Source: CAD feature listing. Evaluate the final solid. Frame: model axes, mm. A direction names the side the tool comes from. Give positions to 0.01 mm unless a question says otherwise; leave off trailing zeros. Loops run counter-clockwise (first coordinate to the right, second up) from the corner with the lowest first, then second, coordinate; pieces in that order, holes last.
Autodesk Inventor part; units mm, degrees
ref_plane "YZ Plane" through (0, 0, 0) normal (1, 0, 0) x (0, 1, 0)
ref_plane "XZ Plane" through (0, 0, 0) normal (0, 1, 0) x (-1, 0, 0)
ref_plane "XY Plane" through (0, 0, 0) normal (0, 0, 1) x (1, 0, 0)
sketch "Esboço1" plane through (0, 0, 0) normal (0, 0, 1) x (1, 0, 0)
  line L0 (0, 0) -> (44, 0)
  line L1 (44, 0) -> (44, 50)
  line L2 (44, 50) -> (0, 50)
  line L3 (0, 50) -> (0, 0)
  dimension "d0" = 44
  dimension "d1" = 50
extrude "Extrusão1" add sketch "Esboço1" along normal blind 3
sketch "Esboço2" plane through (0, 0, 0) normal (-1, 0, 0) x (0, 0, 1)
  line L0 (0, 0) -> (0, 50)
  line L1 (0, 50) -> (-16, 50)
  line L2 (-16, 50) -> (-16, 0)
  line L3 (-16, 0) -> (0, 0)
  line L4 (0, 0) -> (0, 50)
  line L5 (0, 50) -> (-8, 50) construction
  line L6 (-8, 50) -> (-8, 42) construction
  line L7 (0, 0) -> (-8, 0) construction
  line L8 (-8, 0) -> (-8, 8) construction
  circle A0 centre (-8, 42) radius 3
  circle A1 centre (-8, 8) radius 3
  dimension "d4" = 16
  dimension "d5" = 50
  dimension "d6" = 8
  dimension "d7" = 8
  dimension "d8" = 8
  dimension "d9" = 8
  dimension "d10" = 6
  dimension "d11" = 6
extrude "Extrusão2" add sketch "Esboço2" against normal blind 3
sketch "Esboço3" plane through (44, 0, 0) normal (1, 0, 0) x (0, 0, -1)
  line L0 (0, 50) -> (-3, 50)
  line L1 (-3, 50) -> (46, 50)
  line L2 (46, 50) -> (46, 0)
  line L3 (46, 0) -> (-3, 0)
  line L4 (-3, 0) -> (-3, 50)
  point P0 (0, 0)
  dimension "d14" = 49
extrude "Extrusão3" add sketch "Esboço3" along normal blind 3
sketch "Esboço4" plane through (44, 0, -46) normal (0, 0, -1) x (-1, 0, 0)
  line L0 (0, 50) -> (41, 50) construction
  line L1 (0, 50) -> (8, 50) construction
  line L2 (8, 50) -> (8, 42) construction
  line L3 (0, 50) -> (0, 0) construction
  line L4 (0, 0) -> (8, 0) construction
  line L5 (41, 0) -> (0, 0) construction
  line L6 (8, 0) -> (8, 8) construction
  circle A0 centre (8, 42) radius 3
  circle A1 centre (8, 8) radius 3
  line L7 (0, 50) -> (16, 50)
  line L8 (16, 50) -> (16, 42)
  line L9 (16, 42) -> (11, 35.755)
  line L10 (11, 35.755) -> (0, 35.755)
  line L11 (0, 50) -> (0, 35.755)
  line L12 (0, 0) -> (16, 0)
  line L13 (16, 0) -> (16, 8)
  line L14 (16, 8) -> (11, 14.245)
  line L15 (11, 14.245) -> (0, 14.245)
  line L16 (0, 0) -> (0, 14.245)
  point P0 (44, 0)
  dimension "d17" = 8
  dimension "d18" = 8
  dimension "d19" = 8
  dimension "d20" = 8
  dimension "d21" = 6
  dimension "d22" = 6
  dimension "d23" = 16
  dimension "d24" = 8
  dimension "d25" = 8
  dimension "d26" = 8
extrude "Extrusão4" add sketch "Esboço4" against normal blind 3
sketch "Esboço5" plane through (0, 50, -16) normal (0, 1, 0) x (1, 0, 0)
  line L0 (0, 0) -> (0, -19)
  line L1 (47, 30) -> (47, -19)
  line L2 (0, -19) -> (47, -19)
  line L3 (47, -19) -> (47, 30)
  line L4 (47, 30) -> (0, 30)
  line L5 (0, 30) -> (0, -19)
  point P0 (0, -16)
extrude "Extrusão5" add sketch "Esboço5" along normal blind 3
sketch "Esboço6" plane through (0, 0, -16) normal (0, -1, 0) x (1, 0, 0)
  line L0 (47, -30) -> (0, -30)
  line L1 (0, 19) -> (47, 19)
  line L2 (0, -30) -> (47, -30)
  line L3 (47, -30) -> (47, 19)
  line L4 (47, 19) -> (0, 19)
  line L5 (0, 19) -> (0, -30)
  point P0 (0, 16)
extrude "Extrusão6" add sketch "Esboço6" along normal blind 3
sketch "Esboço7" plane through (0, -3, -16) normal (0, -1, 0) x (1, 0, 0)
  point P0 (0, 16)
  point P1 (5.9184, 10.7829)
  point P2 (9.9362, 10.9743)
hole "Furo1" at (5.9184, -3, -5.2171) at (9.9362, -3, -5.0257) direction (0, 1, 0) diameter 2 depth 3 tip angle 118
sketch "Esboço8" plane through (0, -3, -16) normal (0, -1, 0) x (1, 0, 0)
  circle A0 centre (5.9184, 10.7829) radius 1
sketch "Esboço9" plane through (0, -3, -16) normal (0, -1, 0) x (1, 0, 0)
  circle A0 centre (9.9362, 10.9743) radius 1
properties part number "KS diant C" material "Plástico, preto opaco"
(1) Section C-C, the plane y = 48. Return the cut outline in (x, z).
A:
outline: (0, -16) - (3, -16) - (3, 0) - (44, 0) - (44, -43) - (28, -43) - (28, -46) - (47, -46) - (47, 3) - (0, 3) - close
(2) Section B-B, the plane x = 36. Return the cut outline in (y, z) (3 decimals).
A:
outline: (-3, -46) - (5, -46) - (5, -43) - (0, -43) - (0, 0) - (50, 0) - (50, -43) - (45, -43) - (45, -46) - (53, -46) - (53, 3) - (-3, 3) - close; (11, -46) - (14.245, -46) - (14.245, -43) - (11, -43) - close; (35.755, -46) - (39, -46) - (39, -43) - (35.755, -43) - close
(3) Ray query, line 1 along Y through (x, z) = (1.2, -8); line 2 along Y through (x, z) = (7, -43); line 3 along X through (y, z) = (48, -3). Return the intervals inside material, ascending.
A:
line 1: y = -3 to 5, 11 to 39, 45 to 53
line 2: y = -3 to 0, 50 to 53
line 3: x = 0 to 3, 44 to 47
(4) Reachability of faces 5 (the flat face through (44, 25, -23)), 6 (the cylindrical face through (1.48, 8.9, -5.14)), 7 (the cylindrical face through (38.21, 44.03, -44.52)) from +Z, -Z, +X, -X, +Y, -Y: full face, straight path, thin tool, end or side. Return the list, or none.
A:
face 5: none
face 6: -X
face 7: -Z
(5) Section D-D, the plane z = -8. Return the cut outline in (x, y), then the cut area to 3 significant figures.
A:
outline: (0, -3) - (47, -3) - (47, 53) - (0, 53) - (0, 45) - (3, 45) - (3, 50) - (44, 50) - (44, 0) - (3, 0) - (3, 5) - (0, 5) - close; (0, 11) - (3, 11) - (3, 39) - (0, 39) - close
area: 546 mm2
(6) First-contact query: pin 1 (1.5 mm diameter, centred on x = 17, y = 27, fed in from -Z); pin 2 (2.5 mm diameter, centred on y = 46.5, z = -44.5, fed in from -X); pin 3 (1.5 mm diameter, centred on y = 3, z = -38.5, fed in from -X). Flat tips, straight axial feed; report the tip coordinate or a pass-through.
A:
pin 1: stops at z = 0
pin 2: stops at x = 28
pin 3: stops at x = 44
(7) Section A-A, the plane z = -14. Return the cut outline in (x, y), then the cut area to 3 significant figures.
A:
outline: (0, -3) - (47, -3) - (47, 53) - (0, 53) - close; hole (3, 0) - (44, 0) - (44, 50) - (3, 50) - close
area: 582 mm2
(8) Mould query, pull axis X, two halves, no side actions, for faces 1 (the flat face through (28, 46, -45)), 2 (the cylindrical face through (6.527, -1.479, -4.424)), 3 (the flat face through (23, 25, 0)), 4 (the flat face through (23, 25, 3)). Classes: pulls with the +X half, pulls with the -X half, needs draft (parallel to the pull), parting line crosses it, or undercut.
A:
face 1: pulls with the -X half
face 2: undercut
face 3: undercut
face 4: needs draft
